Job drawing, mm, ordinate dimensions from the low corner. One solid piece. A direction names the side the tool comes from. Round coordinates to 2 decimals unless told otherwise and drop trailing zeros. Loops run counter-clockwise (first coordinate to the right, second up) from the corner with the lowest first, then second, coordinate; pieces in that order, holes last. Notation, with made-up numbers: M 61.25,79.25 L 72.25,79.25 A21 cw 72.25,85.25 Z; hole C 0.5,73.25 d5. An arc over 180 degrees is marked long. One line per item, written item: value.
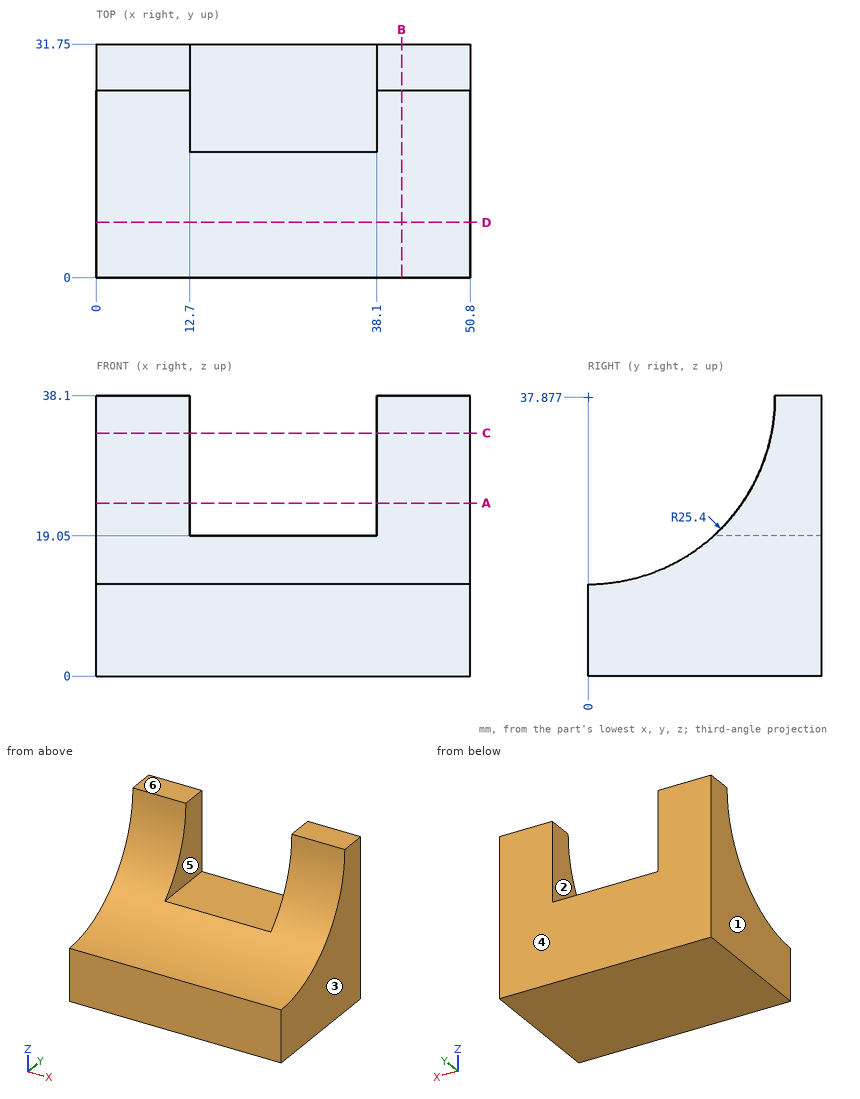
Item 1: Slice it at B-B, the plane x = 41.5. Give the cut face in (y, z), and give its area (3 significant figures).
Check values:
outline: M 0,0 L 31.75,0 L 31.75,38.1 L 25.4,38.1 A25.4 cw 0,12.48 Z
area: 697 mm2
Item 2: Wall check: line 1 along X through (y, z) = (26, 21); line 2 along Z through (x, y) = (27, 27); line 3 along Z through (x, y) = (36, 12). Give the ranges that are in metal, low to high.
Check values:
line 1: x = 0 to 12.7, 38.1 to 50.8
line 2: z = 0 to 19.05
line 3: z = 0 to 15.49
Item 3: Slice it at A-A, the plane z = 23.5. Give the cut face in (x, y).
Check values:
outline: M 0,20.94 L 12.7,20.94 L 12.7,31.75 L 0,31.75 Z; M 38.1,20.94 L 50.8,20.94 L 50.8,31.75 L 38.1,31.75 Z
Item 4: Pull direction X, two halves, no side cores. Call the marked faces 1, 2, 3 and 4: pulls with the +X half, pulls with the -X half, needs draft (parallel to the pull), parting line crosses it, or undercut.
Check values:
face 1: pulls with the -X half
face 2: undercut
face 3: pulls with the +X half
face 4: needs draft
Item 5: Drop flat-ended pins along their axis: P1, Ø16, axis at y = 22, z = 30, coming from the +X side; P2, Ø10, axis at x = 33, y = 7.5, coming from the +Z side; P3, Ø4.5, axis at x = 26, y = 24.5, coming from the +Z side; P4, Ø12, axis at x = 34.5, z = 33.5, coming from the -Y side. Give the stop position or say it passes through.
Check values:
P1: stops at x = 50.8
P2: stops at z = 15.77
P3: stops at z = 19.05
P4: stops at y = 23.68
Item 6: Slice it at C-C, the plane z = 33. Give the cut face in (x, y).
Check values:
outline: M 0,24.93 L 12.7,24.93 L 12.7,31.75 L 0,31.75 Z; M 38.1,24.93 L 50.8,24.93 L 50.8,31.75 L 38.1,31.75 Z
Item 7: Slice it at D-D, the plane y = 7.5. Give the cut face in (x, z), and give its area (3 significant figures).
Check values:
outline: M 0,0 L 50.8,0 L 50.8,13.61 L 0,13.61 Z
area: 691 mm2
Item 8: Which spindle directions (+Z, -Z, +X, -X, +Y, -Y) get a long thin tool onto all of the face, cutting with end or side? Do the marked faces 5 and 6. Say none if no direction does.
Check values:
face 5: +Z, +Y, -Y
face 6: +Z, +X, -X, +Y, -Y
